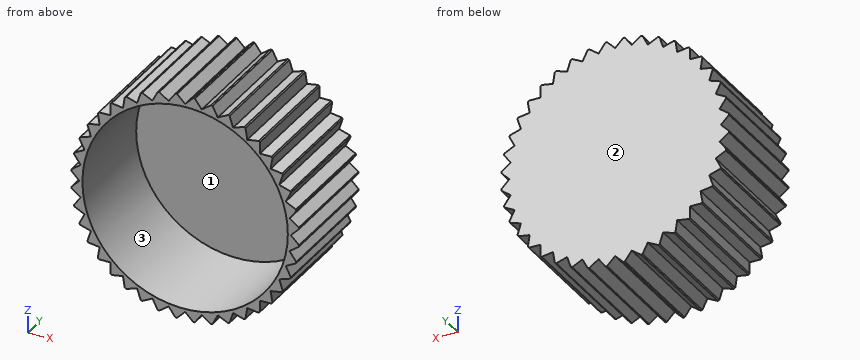
from build123d import *

# Parameters (mm, degrees)
F0_R            = 25.4
F1_DEPTH        = 25.4
F2_T            = -2.54
F6_DEPTH        = 25.4
F6_COPIES_COUNT = 40


# Not quite as in the source:
# - a pattern or mirror of a feature is missing from the dataset's text; its kind, count and spacing are read off the source's solid
# - a feature names something its author has since deleted; it is built from what else it names


with BuildPart() as f1:
    # F0 (on Front) → F1 (new body)
    with BuildSketch(Plane.XZ):
        Circle(F0_R)
    extrude(amount=F1_DEPTH)

    # F2
    f2_openings = [f1.faces().sort_by_distance(p)[0] for p in [
        (0, -25.4, 0),
    ]]
    offset(amount=F2_T, openings=f2_openings)

    # F4 (on offset) → F6 (cut)
    with BuildSketch(Plane.XZ.offset(25.4)):
        Polygon((1.9352714298, 25.4522323095), (-1.9276905805, 25.4598131588), (0, 23.524541729), align=None)
    f6 = extrude(amount=-F6_DEPTH, mode=Mode.SUBTRACT)

    # F6_copies: F6 ×40 about axis
    f6_copies_axis = Axis((0, 0, 0), (0, 1, 0))
    for i in range(1, F6_COPIES_COUNT):
        add(f6.rotate(f6_copies_axis, i * 360 / F6_COPIES_COUNT), mode=Mode.SUBTRACT)


solid = f1.part
Build history of the part. All positions in model axes, mm. Face numbers are marked on the shaded views. Round coordinates to 2 decimals unless told otherwise and drop trailing zeros. Loops run counter-clockwise (first coordinate to the right, second up) from the corner with the lowest first, then second, coordinate; pieces in that order, holes last. Notation, with made-up numbers: (-21.5, -0.75) -> (-7.5, -0.75) arc R22 ccw to (-7.5, 22.25) -> close; hole circle Ø5 at (58, 31). An arc over 180 degrees is marked (long way). Use CSV: the item, a comma, the result in double quotes. Start each with the question number.
Q1. Flat gauge pins, fed straight in: pin 1 Ø5 at (x, y) = (14, -13.5) entering from +Z; pin 2 Ø3 at (y, z) = (-7, 10) entering from -X; pin 3 Ø4 at (y, z) = (-8.5, 12.5) entering from +X. Where does each tip first touch, or does it go through?
Q2. Drill centre lines: L1, parallel to Z at x = 23, y = -19.5; L2, parallel to X at y = -20.5, z = 18.5; L3, parallel to Y at x = -18, z = -1.5. Where is each one in solid material? Low to high.
Q3. Saw through at B-B on z = 1. Give the cut face in (x, y).
Q4. Saw through at A-A on x = -1. Give the cut face in (y, z).
Q5. Mould opens along Z. For the marked faces 1, 2 and 3 say: +Z half, -Z half, draft (parallel to the pull), parting line (faces both ways), or undercut.
Solutions:
1,pin 1,"stops at z = 21.75"
1,pin 2,"stops at x = -23.53"
1,pin 3,"stops at x = 21.76"
2,L1,"z = -10.02 to -8.51, -6.95 to 6.95, 8.49 to 10.01"
2,L2,"x = -16.63 to -13.43, 13.43 to 16.64"
2,L3,"y = -2.54 to 0"
3,outline,"(-24.52, -25.4) -> (-22.84, -25.4) -> (-22.84, -2.54) -> (22.84, -2.54) -> (22.84, -25.4) -> (24.53, -25.4) -> (24.53, 0) -> (-24.52, 0) -> close"
4,outline,"(-25.4, -24.52) -> (0, -24.52) -> (0, 24.53) -> (-25.4, 24.53) -> (-25.4, 22.84) -> (-2.54, 22.84) -> (-2.54, -22.84) -> (-25.4, -22.84) -> close"
5,face 1,"undercut"
5,face 2,"draft"
5,face 3,"undercut"
